```python
from build123d import *

# Parameters (mm, degrees)
F0_W      = 76.2
F0_H      = 76.2
F1_DEPTH  = 19.05
F2_R      = 19.05
F3_DEPTH  = 25.4
F4_R      = 19.05
F5_DEPTH  = 50.8
F6_W      = 76.2
F6_H      = 76.2
F7_DEPTH  = 19.05
F8_R      = 25.4
F9_DEPTH  = 76.2
F10_R     = 19.05
F11_DEPTH = 114.3
F12_R     = 6.35
F14_DEPTH = 114.3
F13_R     = 6.5396642154
F13_R_2   = 6.35
F15_DEPTH = 127


with BuildPart() as f1:
    # F0 (on Front) → F1 (new body)
    with BuildSketch(Plane.XZ):
        Rectangle(F0_W, F0_H)
    extrude(amount=F1_DEPTH)

    # F2 (on face) → F3 (join)
    with BuildSketch(Plane.XZ.offset(19.05)):
        Circle(F2_R)
    extrude(amount=F3_DEPTH)

    # F4 (on face) → F5 (join)
    with BuildSketch(Plane.XZ.offset(44.45)):
        Circle(F4_R)
    extrude(amount=F5_DEPTH)

    # F6 (on face) → F7 (join)
    with BuildSketch(Plane.XZ.offset(95.25)):
        Rectangle(F6_W, F6_H)
    extrude(amount=F7_DEPTH)

    # F8 (on face) → F9 (join)
    with BuildSketch(Plane(origin=(0, -95.25, 0), x_dir=(-1, 0, 0), z_dir=(0, 1, 0))):
        Circle(F8_R)
    extrude(amount=F9_DEPTH)

    # F10 (on face) → F11 (cut)
    with BuildSketch(Plane(origin=(0, 0, 0), x_dir=(-1, 0, 0), z_dir=(0, 1, 0))):
        Circle(F10_R)
    extrude(amount=-F11_DEPTH, mode=Mode.SUBTRACT)

    # F12 (on face) → F14 (cut)
    with BuildSketch(Plane(origin=(0, 0, 0), x_dir=(-1, 0, 0), z_dir=(0, 1, 0))):
        with Locations((25.5859810859, 27.2544045001)):
            Circle(F12_R)
    extrude(amount=-F14_DEPTH, mode=Mode.SUBTRACT)

    # F13 (on face) → F15 (cut)
    with BuildSketch(Plane(origin=(0, 0, 0), x_dir=(-1, 0, 0), z_dir=(0, 1, 0))):
        with Locations((-27.4109728634, 29.1734542698)):
            Circle(F13_R)
        with Locations((-26.7679095268, -28.0488487333)):
            Circle(F13_R_2)
        with Locations((26.6334090033, -27.1274481038)):
            Circle(F13_R_2)
    extrude(amount=-F15_DEPTH, mode=Mode.SUBTRACT)


solid = f1.part
```
Geometry check sheet. Reference: the model listing, model coordinates, mm. A direction names the side the tool comes from. Give positions to 0.01 mm unless a question says otherwise; leave off trailing zeros. Order: outer loops, then holes, each group sorted by start corner. A loop starts at its lowest first (then second) coordinate and runs counter-clockwise, first axis right, second up. Notation, with made-up numbers: (33.5, -23) - (77.5, -23) arc R28 cw to (77.5, 3) - close; hole circle Ø7 at (47, 14.5). An arc over 180 degrees is marked (long way). Write item = value, one per line. Start each with the question number.
1) Section check D-D (x = -28). Enter the section's corners in (y, z), then the cut area to 3 significant figures.
2) Section check C-C (y = -14). Enter the section's corners in (x, z).
3) Draft check along X on faces 3 (the cylindrical face through (-32.69, -104.64, -25.22)), 4 (the cylindrical face through (-24.209, -9.392, 21.055)), 5 (the flat face through (-1, -105, -38.1)), 6 (the flat face through (-38.1, -105, -1)). Enter one of: released by +X, released by -X, zero draft, split by the parting line, or undercut.
4) Gauge pin test, flat ends, axial feed: pin 1 Ø11.5 at (x, z) = (-25.59, 27.25) entering from +Y; pin 2 Ø1.5 at (y, z) = (-77.5, -15) entering from -X; pin 3 Ø1.5 at (x, y) = (0.5, -53) entering from +Z. Record the tip position at first contact, or that the pin passes through.
5) Section check B-B (z = 0). Enter the section's corners in (x, y), then the cut area to 3 significant figures.
6) Access from +Z, -Z, +X, -X, +Y, -Y to the whole of each face (thin tool, end or side, straight path). Record for faces 1 (the flat face through (-9, -114.3, 17)), 2 (the flat face through (-1, -19.05, 26)).
7) Section check A-A (x = 0). Enter the section's corners in (y, z).
8) Scan lines: L1, parallel to X at y = -51, z = 0.5; L2, parallel to Y at x = 32.5, z = 35; L3, parallel to Z at x = 29, y = -5. Record each from-to range of solid material in increasing order.
Geometry check:
q1.outline = (-114.3, -38.1) - (-95.25, -38.1) - (-95.25, -33.33) - (-114.3, -33.33) - close; (-114.3, -20.93) - (-95.25, -20.93) - (-95.25, 21.38) - (-114.3, 21.38) - close; (-114.3, 33.13) - (-95.25, 33.13) - (-95.25, 38.1) - (-114.3, 38.1) - close; (-19.05, -38.1) - (0, -38.1) - (0, -33.33) - (-19.05, -33.33) - close; (-19.05, -20.93) - (0, -20.93) - (0, 21.38) - (-19.05, 21.38) - close; (-19.05, 33.13) - (0, 33.13) - (0, 38.1) - (-19.05, 38.1) - close
q1.area = 1,980 mm2
q2.outline = (-38.1, -38.1) - (38.1, -38.1) - (38.1, 38.1) - (-38.1, 38.1) - close; hole circle Ø12.7 at (-26.63, -27.13); hole circle Ø12.7 at (-25.59, 27.25); hole circle Ø38.1 at (0, 0); hole circle Ø12.7 at (26.77, -28.05); hole circle Ø13.08 at (27.41, 29.17)
q3.face_3 = undercut
q3.face_4 = undercut
q3.face_5 = zero draft
q3.face_6 = released by -X
q4.pin_1 = through
q4.pin_2 = -21.03
q4.pin_3 = 25.4
q5.outline = (-38.1, -114.3) - (-19.05, -114.3) - (-19.05, 0) - (-38.1, 0) - (-38.1, -19.05) - (-25.4, -19.05) - (-25.4, -95.25) - (-38.1, -95.25) - close; (19.05, -114.3) - (38.1, -114.3) - (38.1, -95.25) - (25.4, -95.25) - (25.4, -19.05) - (38.1, -19.05) - (38.1, 0) - (19.05, 0) - close
q5.area = 2,420 mm2
q6.face_1 = +Z, -Z, +X, -X, -Y
q6.face_2 = none
q7.outline = (-114.3, -38.1) - (-95.25, -38.1) - (-95.25, -25.4) - (-19.05, -25.4) - (-19.05, -38.1) - (0, -38.1) - (0, -19.05) - (-114.3, -19.05) - close; (-114.3, 19.05) - (0, 19.05) - (0, 38.1) - (-19.05, 38.1) - (-19.05, 25.4) - (-95.25, 25.4) - (-95.25, 38.1) - (-114.3, 38.1) - close
q8.L1 = -25.4 to -19.04, 19.04 to 25.4
q8.L2 = -114.3 to -95.25, -19.05 to 0
q8.L3 = -38.1 to -33.99, -22.1 to 22.83, 35.52 to 38.1
